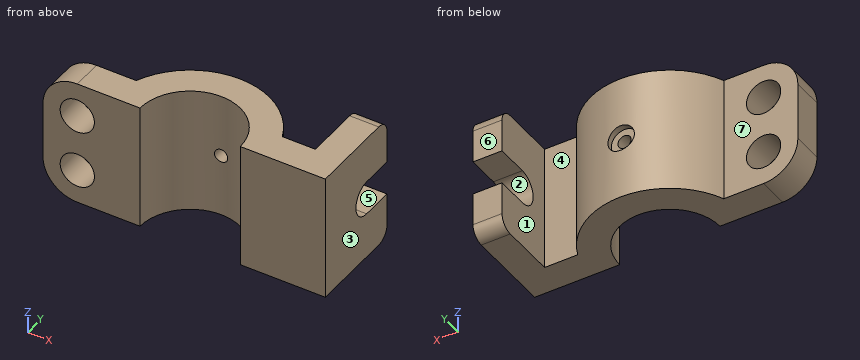
```python
from build123d import *

# Parameters (mm, degrees)
F1_DEPTH        = 48
F2_R            = 5
F4_DEPTH        = 11
F5_R            = 13
F6_R            = 6.5
F7_DEPTH        = 25
F10_D           = 5
F10_START       = 0.4342628
F10_CBORE_D     = 10
F10_CBORE_DEPTH = 2


with BuildPart() as f1:
    # F0 (on Top) → F1 (new body)
    with BuildSketch(Plane.XY):
        with BuildLine():
            Line((-8.6803510502, 11.5671157052), (-36.7703510502, 11.5671157052))
            Line((-36.7703510502, 11.5671157052), (-36.7703510502, 0))
            Line((-36.7703510502, 0), (0, 0))
            ThreePointArc((0, 0), (19, 19), (38, 0))
            Line((38, 0), (70.2296489498, 0))
            Line((70.2296489498, 0), (70.2296489498, 37.3193000675))
            Line((70.2296489498, 37.3193000675), (59.2296489498, 37.3193000675))
            Line((59.2296489498, 37.3193000675), (59.2296489498, 11.5671157052))
            Line((59.2296489498, 11.5671157052), (46.6803510502, 11.5671157052))
            ThreePointArc((46.6803510502, 11.5671157052), (19, 30), (-8.6803510502, 11.5671157052))
        make_face()
    extrude(amount=F1_DEPTH)

    # F2
    f2_edges = [f1.edges().sort_by_distance(p)[0] for p in [
        (64.729649, 37.3193, 48),
        (64.729649, 37.3193, 0),
    ]]
    fillet(f2_edges, radius=F2_R)

    # F3 (on face) → F4 (cut)
    with BuildSketch(Plane.YZ.offset(70.2296489498)):
        with BuildLine():
            Line((37.3193000675, 17.5), (37.3193000675, 30.5))
            Line((37.3193000675, 30.5), (25, 30.5))
            ThreePointArc((25, 30.5), (18.5, 24), (25, 17.5))
            Line((25, 17.5), (37.3193000675, 17.5))
        make_face()
    extrude(amount=-F4_DEPTH, mode=Mode.SUBTRACT)

    # F5
    f5_edges = [f1.edges().sort_by_distance(p)[0] for p in [
        (-36.770351, 5.783558, 48),
        (-36.770351, 5.783558, 0),
    ]]
    fillet(f5_edges, radius=F5_R)

    # F6 (on face) → F7 (cut)
    with BuildSketch(Plane(origin=(0, 11.5671157052, 0), x_dir=(-1, 0, 0), z_dir=(0, 1, 0))):
        with Locations((23.7703510502, 13)):
            Circle(F6_R)
        with Locations((23.7703510502, 35)):
            Circle(F6_R)
    extrude(amount=-F7_DEPTH, mode=Mode.SUBTRACT)

    # F10 (through all)
    # its depths count from where the whole tool has entered the part; down to there all is cleared
    with Locations(Plane(origin=(0, 30, 0), x_dir=(1, 0, 0), z_dir=(0, 1, 0)).offset(-F10_START)):
        with Locations((18.9140215516, -23.9382665604)):
            CounterBoreHole(F10_D / 2, F10_CBORE_D / 2, F10_CBORE_DEPTH)


solid = f1.part
```
Model file for the job. Use its own axes, mm. Face numbers are marked on the shaded views. A direction names the side the tool comes from. Round coordinates to 2 decimals unless told otherwise and drop trailing zeros. Order: outer loops, then holes, each group sorted by start corner. A loop starts at its lowest first (then second) coordinate and runs counter-clockwise, first axis right, second up. Notation, with made-up numbers: (-12, 44.5) -> (-1, 44.5) arc R9 cw to (-1, 49.5) -> close; hole circle Ø2 at (58.5, 15). An arc over 180 degrees is marked (long way). Use one line per item in the form item = value.
Item 1: Cut at D-D, the plane x = -26. Write the cut outline in (y, z).
Returned:
outline = (0, 0.19) -> (11.57, 0.19) -> (11.57, 6.89) -> (0, 6.89) -> close; (0, 19.11) -> (11.57, 19.11) -> (11.57, 28.89) -> (0, 28.89) -> close; (0, 41.11) -> (11.57, 41.11) -> (11.57, 47.81) -> (0, 47.81) -> close
Item 2: Cut at B-B, the plane x = 19. Write the cut outline in (y, z), and give its area (3 significant figures).
Returned:
outline = (19, 0) -> (30, 0) -> (30, 18.94) -> (27.57, 18.94) -> (27.57, 21.44) -> (19, 21.44) -> close; (19, 26.44) -> (27.57, 26.44) -> (27.57, 28.94) -> (30, 28.94) -> (30, 48) -> (19, 48) -> close
area = 461 mm^2
Item 3: Flat gauge pins, fed straight in: pin 1 Ø5 at (x, z) = (18, 9.5) entering from +Y; pin 2 Ø10 at (x, z) = (51, 14.5) entering from +Y; pin 3 Ø9 at (x, z) = (18.91, 23.94) entering from +Y; pin 4 Ø10.5 at (x, z) = (-23.77, 13) entering from +Y. Where does each tip first touch, or does it go through?
Returned:
pin_1 = 30
pin_2 = 13.08
pin_3 = 27.57
pin_4 = through
Item 4: Cut at C-C, the plane y = 21.5. Write the cut outline in (x, z).
Returned:
outline = (-1.92, 0) -> (39.92, 0) -> (39.92, 48) -> (-1.92, 48) -> close; (59.23, 0) -> (70.23, 0) -> (70.23, 18.52) -> (59.23, 18.52) -> close; (59.23, 29.48) -> (70.23, 29.48) -> (70.23, 48) -> (59.23, 48) -> close; hole circle Ø5 at (18.91, 23.94)
Item 5: Tool access for the marked faces 4, 5, 6 and 7: list every direction of +Z, -Z, +X, -X, +Y, -Y with a clear straight run to the whole face (end or side of a thin tool).
Returned:
face_4 = +Z, -Z, +Y
face_5 = +X, +Y
face_6 = +Z, -Z, +X, -X, +Y
face_7 = +Z, -Z, -X, +Y
Item 6: Drill centre lines: line 1 (Z direction, x = 65, y = 27); line 2 (X direction, y = 17.5, z = 38); line 3 (X direction, y = 6, z = 36). Where is each one in solid material? Low to high.
Returned:
line_1 = 0 to 17.5, 30.5 to 48
line_2 = -5.37 to 11.6, 26.4 to 43.37, 59.23 to 70.23
line_3 = -36.73 to -30.19, -17.35 to 0.97, 37.03 to 70.23
Item 7: Cut at A-A, the plane y = 6. Write the cut outline in (x, z), and give its area (3 significant figures).
Returned:
outline = (-36.77, 13) arc R13 ccw to (-23.77, 0) -> (0.97, 0) -> (0.97, 48) -> (-23.77, 48) arc R13 ccw to (-36.77, 35) -> close; (37.03, 0) -> (70.23, 0) -> (70.23, 48) -> (37.03, 48) -> close; hole circle Ø13 at (-23.77, 13); hole circle Ø13 at (-23.77, 35)
area = 3,070 mm^2
Item 8: Pull direction X, two halves, no side cores. Call the marked faces 1, 2 and 3: released by +X, released by -X, zero draft, split by the parting line, or undercut.
Returned:
face_1 = undercut
face_2 = zero draft
face_3 = released by +X
